Can you work these out from the model? Positions are in its coordinate system, mm. A direction names the side the tool comes from. Coordinates: 2 decimals unless noted, no trailing zeros. Write each loop counter-clockwise with the first axis right and the second up, starting at its lowest first coordinate (ties: lowest second). Pieces come first, ordered by that corner, then holes.
```python
from build123d import *

# Parameters (mm, degrees)
F0_R     = 1.6
F1_DEPTH = 52
F2_DEPTH = 2
F4_DEPTH = 2
F5_R     = 2


with BuildPart() as f1:
    # F0 (on Top) → F1 (new body)
    with BuildSketch(Plane.XY):
        Polygon((22.3549354323, 10), (22.3549354323, 11.5), (-7.6450645677, 11.5), (-7.6450645677, -18.5), (-6.1450645677, -18.5), (-6.1450645677, -3.5), (-2.6450645677, -3.5), (-2.6450645677, -18.5), (-1.1450645677, -18.5), (-1.1450645677, 0), (-1.1450645677, 5), (3.8549354323, 5), (22.3549354323, 5), (22.3549354323, 6.5), (7.3549354323, 6.5), (7.3549354323, 10), align=None)
        with Locations((-4.0450645677, 7.9)):
            Circle(F0_R, mode=Mode.SUBTRACT)
    extrude(amount=F1_DEPTH)

    # F0 (on Top) → F2 (join)
    with BuildSketch(Plane.XY):
        Polygon((-1.1450645677, 0), (3.8549354323, 5), (-1.1450645677, 5), align=None)
    extrude(amount=F2_DEPTH)

    # F3 (on face) → F4 (join)
    with BuildSketch(Plane.XY.offset(52)):
        Polygon((-1.1450645677, 0), (3.8549354323, 5), (-1.1450645677, 5), align=None)
    extrude(amount=-F4_DEPTH)

    # F5
    f5_edges = [f1.edges().sort_by_distance(p)[0] for p in [
        (-1.145065, 5, 26),
        (3.854935, 5, 1),
        (-1.145065, 0, 1),
        (-1.145065, 0, 51),
        (3.854935, 5, 51),
        (-7.645065, 11.5, 26),
    ]]
    fillet(f5_edges, radius=F5_R)


solid = f1.part
```
1. If we section it at A-A, the plane y = -9.5: List the corners of the cut face in (x, z) for me, plus the area to 3 significant figures.
2. If we section it at B-B, the plane z = 4.5: List the corners of the cut face in (x, y) for me.
3. I'm going to push flat-ended pins straight in: P1, Ø12, axis at x = 18.5, z = 26, coming from the -Y side; P2, Ø1, axis at x = -4.5, z = 35, coming from the -Y side; P3, Ø7.5, axis at y = -14, z = 30, coming from the +X side; P4, Ø1.7, axis at x = 2.5, y = 1.5, coming from the -Z side. Where does each tip first touch, or does it pass through?
4. Which directions (+Z, -Z, +X, -X, +Y, -Y) give clear straight access to the entire face, cutting with the end or side of a thin tool? Please do faces 1 (the face through (11, 5, 26)), 2 (the face through (15, 6.5, 26)), 3 (the face through (-5.224, 8.981, 25.636)), 4 (the face through (-4, -3.5, 26)).
5. If we section it at D-D, the plane x = 1.5: List the corners of the cut face in (y, z) for me.
6. If we section it at C-C, the plane x = 13.25: List the corners of the cut face in (y, z) for me, plus the area to 3 significant figures.
7. If I drill on L1, parallel to X at y = -16.25, z = 23; L2, parallel to Y at x = 14, z = 17; L3, parallel to X at y = -3.25, z = 37, over which ranges is the centre line in solid material (lowest first)?
8. We'd pull the mould along Z, two halves only. Please class faces 5 (the face through (3.908, 4.844, 50.986)), 6 (the face through (-0.575, 4.399, 26.336)), 7 (the face through (1, 3, 0)): released by +Z, released by -Z, zero draft, split by the parting line, or undercut.
Answers:
1. outline: (-7.65, 0) - (-6.15, 0) - (-6.15, 52) - (-7.65, 52) - close; (-2.65, 0) - (-1.15, 0) - (-1.15, 52) - (-2.65, 52) - close
1. area: 156 mm2
2. outline: (-7.65, -18.5) - (-6.15, -18.5) - (-6.15, -3.5) - (-2.65, -3.5) - (-2.65, -18.5) - (-1.15, -18.5) - (-1.15, 3) arc R2 cw to (0.85, 5) - (22.35, 5) - (22.35, 6.5) - (7.35, 6.5) - (7.35, 10) - (22.35, 10) - (22.35, 11.5) - (-5.65, 11.5) arc R2 ccw to (-7.65, 9.5) - close; hole circle Ø3.2 at (-4.05, 7.9)
3. P1: stops at y = 5
3. P2: stops at y = -3.5
3. P3: stops at x = -1.15
3. P4: passes through
4. face 1: +X, -Y
4. face 2: +Z, -Z, +X
4. face 3: +Z, -Z
4. face 4: +Z, -Z, -Y
5. outline: (2.65, 0) - (11.5, 0) - (11.5, 52) - (2.65, 52) - (2.65, 50) - (5, 50) - (5, 2) - (2.65, 2) - close
6. outline: (5, 0) - (6.5, 0) - (6.5, 52) - (5, 52) - close; (10, 0) - (11.5, 0) - (11.5, 52) - (10, 52) - close
6. area: 156 mm2
7. L1: x = -7.65 to -6.15, -2.65 to -1.15
7. L2: y = 5 to 6.5, 10 to 11.5
7. L3: x = -7.65 to -1.15
8. face 5: zero draft
8. face 6: undercut
8. face 7: released by -Z
